Build history of the part. All positions in model axes, mm. A direction names the side the tool comes from. Give positions to 0.01 mm unless a question says otherwise; leave off trailing zeros. Order: outer loops, then holes, each group sorted by start corner. A loop starts at its lowest first (then second) coordinate and runs counter-clockwise, first axis right, second up. Notation, with made-up numbers: (1, 34.5) - (19, 34.5) arc R15 cw to (19, 57.5) - close; hole circle Ø6 at (79, -32). An arc over 180 degrees is marked (long way). Answer in a Markdown table with one row per item.
```python
from build123d import *

# Parameters (mm, degrees)
BOSS_EXTRUDE1_DEPTH = 206
SKETCH2_W           = 10
SKETCH2_H           = 6
BOSS_EXTRUDE2_DEPTH = 10
CUT_EXTRUDE1_REACH  = 202
SKETCH3_R           = 1.5
CUT_EXTRUDE2_REACH  = 33.335
SKETCH4_R           = 2
CUT_EXTRUDE3_REACH  = 33.335
SKETCH5_R           = 1.5
CUT_EXTRUDE4_REACH  = 33.335
SKETCH6_R           = 1.5
CUT_EXTRUDE5_REACH  = 103.569
SKETCH7_R           = 1.5
CUT_EXTRUDE6_REACH  = 103.569
SKETCH8_R           = 1.5


with BuildPart() as part:
    # Sketch1 → Boss-Extrude1 (new body)
    with BuildSketch(Plane(origin=(0, 0, 0), x_dir=(1, 0, 0), z_dir=(0, 1, 0))):
        Polygon((-40, 0), (40, 0), (63.334523779, 23.334523779), (68.991378029, 17.67766953), (43.313708499, -8), (-43.313708499, -8), (-68.991378029, 17.67766953), (-63.334523779, 23.334523779), align=None)
    extrude(amount=BOSS_EXTRUDE1_DEPTH)

    # Sketch2 → Boss-Extrude2 (add)
    with BuildSketch(Plane(origin=(0, 0, 0), x_dir=(-1, 0, 0), z_dir=(0, 0, -1))):
        with Locations((-29, 197)):
            Rectangle(SKETCH2_W, SKETCH2_H)
        with Locations((29, 197)):
            Rectangle(SKETCH2_W, SKETCH2_H)
    extrude(amount=BOSS_EXTRUDE2_DEPTH)

    # Sketch3 → Cut-Extrude1 (cut, up to next)
    with BuildSketch(Plane(origin=(0, 200, 0), x_dir=(1, 0, 0), z_dir=(0, 1, 0)), mode=Mode.PRIVATE) as cut_extrude1_sk1:
        with Locations((-29, 5)):
            Circle(SKETCH3_R)
    cut_extrude1_tool1 = extrude(cut_extrude1_sk1.sketch, amount=-CUT_EXTRUDE1_REACH, mode=Mode.PRIVATE) & part.part
    add(cut_extrude1_tool1.solids().sort_by_distance((-29, 200, -5))[0], mode=Mode.SUBTRACT)
    # Sketch3 → Cut-Extrude1 (cut, up to next)
    with BuildSketch(Plane(origin=(0, 200, 0), x_dir=(1, 0, 0), z_dir=(0, 1, 0)), mode=Mode.PRIVATE) as cut_extrude1_sk2:
        with Locations((29, 5)):
            Circle(SKETCH3_R)
    cut_extrude1_tool2 = extrude(cut_extrude1_sk2.sketch, amount=-CUT_EXTRUDE1_REACH, mode=Mode.PRIVATE) & part.part
    add(cut_extrude1_tool2.solids().sort_by_distance((29, 200, -5))[0], mode=Mode.SUBTRACT)

    # Sketch4 → Cut-Extrude2 (cut, up to next)
    with BuildSketch(Plane.XY.offset(8), mode=Mode.PRIVATE) as cut_extrude2_sk1:
        with Locations((-14.667053615, 27)):
            Circle(SKETCH4_R)
    cut_extrude2_tool1 = extrude(cut_extrude2_sk1.sketch, amount=-CUT_EXTRUDE2_REACH, mode=Mode.PRIVATE) & part.part
    add(cut_extrude2_tool1.solids().sort_by_distance((-14.667054, 27, 8))[0], mode=Mode.SUBTRACT)
    # Sketch4 → Cut-Extrude2 (cut, up to next)
    with BuildSketch(Plane.XY.offset(8), mode=Mode.PRIVATE) as cut_extrude2_sk2:
        with Locations((11.313708499, 12)):
            Circle(SKETCH4_R)
    cut_extrude2_tool2 = extrude(cut_extrude2_sk2.sketch, amount=-CUT_EXTRUDE2_REACH, mode=Mode.PRIVATE) & part.part
    add(cut_extrude2_tool2.solids().sort_by_distance((11.313708, 12, 8))[0], mode=Mode.SUBTRACT)

    # Sketch5 → Cut-Extrude3 (cut, up to next)
    with BuildSketch(Plane.XY.offset(8), mode=Mode.PRIVATE) as cut_extrude3_sk1:
        with Locations((-7, 76.404082058)):
            Circle(SKETCH5_R)
    cut_extrude3_tool1 = extrude(cut_extrude3_sk1.sketch, amount=-CUT_EXTRUDE3_REACH, mode=Mode.PRIVATE) & part.part
    add(cut_extrude3_tool1.solids().sort_by_distance((-7, 76.404082, 8))[0], mode=Mode.SUBTRACT)
    # Sketch5 → Cut-Extrude3 (cut, up to next)
    with BuildSketch(Plane.XY.offset(8), mode=Mode.PRIVATE) as cut_extrude3_sk2:
        with Locations((7, 76.404082058)):
            Circle(SKETCH5_R)
    cut_extrude3_tool2 = extrude(cut_extrude3_sk2.sketch, amount=-CUT_EXTRUDE3_REACH, mode=Mode.PRIVATE) & part.part
    add(cut_extrude3_tool2.solids().sort_by_distance((7, 76.404082, 8))[0], mode=Mode.SUBTRACT)

    # Sketch6 → Cut-Extrude4 (cut, up to next)
    with BuildSketch(Plane.XY.offset(8), mode=Mode.PRIVATE) as cut_extrude4_sk1:
        with Locations((-25.813708499, 171)):
            Circle(SKETCH6_R)
    cut_extrude4_tool1 = extrude(cut_extrude4_sk1.sketch, amount=-CUT_EXTRUDE4_REACH, mode=Mode.PRIVATE) & part.part
    add(cut_extrude4_tool1.solids().sort_by_distance((-25.813708, 171, 8))[0], mode=Mode.SUBTRACT)
    # Sketch6 → Cut-Extrude4 (cut, up to next)
    with BuildSketch(Plane.XY.offset(8), mode=Mode.PRIVATE) as cut_extrude4_sk2:
        with Locations((25.813708499, 171)):
            Circle(SKETCH6_R)
    cut_extrude4_tool2 = extrude(cut_extrude4_sk2.sketch, amount=-CUT_EXTRUDE4_REACH, mode=Mode.PRIVATE) & part.part
    add(cut_extrude4_tool2.solids().sort_by_distance((25.813708, 171, 8))[0], mode=Mode.SUBTRACT)
    # Sketch6 → Cut-Extrude4 (cut, up to next)
    with BuildSketch(Plane.XY.offset(8), mode=Mode.PRIVATE) as cut_extrude4_sk3:
        with Locations((-25.813708499, 106)):
            Circle(SKETCH6_R)
    cut_extrude4_tool3 = extrude(cut_extrude4_sk3.sketch, amount=-CUT_EXTRUDE4_REACH, mode=Mode.PRIVATE) & part.part
    add(cut_extrude4_tool3.solids().sort_by_distance((-25.813708, 106, 8))[0], mode=Mode.SUBTRACT)
    # Sketch6 → Cut-Extrude4 (cut, up to next)
    with BuildSketch(Plane.XY.offset(8), mode=Mode.PRIVATE) as cut_extrude4_sk4:
        with Locations((25.813708499, 89)):
            Circle(SKETCH6_R)
    cut_extrude4_tool4 = extrude(cut_extrude4_sk4.sketch, amount=-CUT_EXTRUDE4_REACH, mode=Mode.PRIVATE) & part.part
    add(cut_extrude4_tool4.solids().sort_by_distance((25.813708, 89, 8))[0], mode=Mode.SUBTRACT)

    # Sketch7 → Cut-Extrude5 (cut, up to next)
    with BuildSketch(Plane(origin=(-25.656854249, 0, 25.656854249), x_dir=(0.707106781, 0, 0.707106781), z_dir=(-0.707106781, 0, 0.707106781)), mode=Mode.PRIVATE) as cut_extrude5_sk1:
        with Locations((-43.414271247, 171)):
            Circle(SKETCH7_R)
    cut_extrude5_tool1 = extrude(cut_extrude5_sk1.sketch, amount=-CUT_EXTRUDE5_REACH, mode=Mode.PRIVATE) & part.part
    add(cut_extrude5_tool1.solids().sort_by_distance((-56.35538, 171, -5.041671))[0], mode=Mode.SUBTRACT)
    # Sketch7 → Cut-Extrude5 (cut, up to next)
    with BuildSketch(Plane(origin=(-25.656854249, 0, 25.656854249), x_dir=(0.707106781, 0, 0.707106781), z_dir=(-0.707106781, 0, 0.707106781)), mode=Mode.PRIVATE) as cut_extrude5_sk2:
        with Locations((-43.414271247, 81)):
            Circle(SKETCH7_R)
    cut_extrude5_tool2 = extrude(cut_extrude5_sk2.sketch, amount=-CUT_EXTRUDE5_REACH, mode=Mode.PRIVATE) & part.part
    add(cut_extrude5_tool2.solids().sort_by_distance((-56.35538, 81, -5.041671))[0], mode=Mode.SUBTRACT)

    # Sketch8 → Cut-Extrude6 (cut, up to next)
    with BuildSketch(Plane(origin=(25.656854249, 0, 25.656854249), x_dir=(0.707106781, 0, -0.707106781), z_dir=(0.707106781, 0, 0.707106781)), mode=Mode.PRIVATE) as cut_extrude6_sk1:
        with Locations((40.384271247, 171)):
            Circle(SKETCH8_R)
    cut_extrude6_tool1 = extrude(cut_extrude6_sk1.sketch, amount=-CUT_EXTRUDE6_REACH, mode=Mode.PRIVATE) & part.part
    add(cut_extrude6_tool1.solids().sort_by_distance((54.212846, 171, -2.899138))[0], mode=Mode.SUBTRACT)
    # Sketch8 → Cut-Extrude6 (cut, up to next)
    with BuildSketch(Plane(origin=(25.656854249, 0, 25.656854249), x_dir=(0.707106781, 0, -0.707106781), z_dir=(0.707106781, 0, 0.707106781)), mode=Mode.PRIVATE) as cut_extrude6_sk2:
        with Locations((40.384271247, 76)):
            Circle(SKETCH8_R)
    cut_extrude6_tool2 = extrude(cut_extrude6_sk2.sketch, amount=-CUT_EXTRUDE6_REACH, mode=Mode.PRIVATE) & part.part
    add(cut_extrude6_tool2.solids().sort_by_distance((54.212846, 76, -2.899138))[0], mode=Mode.SUBTRACT)


solid = part.part
```
1. Cut at D-D on x = -46.5. Write the cut outline in (y, z).
Check result:
| item | result |
|---|---|
| outline | (0, -6.5) - (206, -6.5) - (206, 4.81) - (0, 4.81) - close |
2. Drop flat-ended pins along their axis: P1, Ø4, axis at y = 35, z = 4, coming from the +X side; P2, Ø10, axis at y = 27, z = 2, coming from the +X side; P3, Ø6.5, axis at x = -14.67, y = 27, coming from the -Z side; P4, Ø3.5, axis at x = 25.81, y = 89, coming from the +Z side. Give the stop position or say it passes through.
Check result:
| item | result |
|---|---|
| P1 | stops at x = 49.31 |
| P2 | stops at x = 54.31 |
| P3 | stops at z = 0 |
| P4 | stops at z = 8 |
3. Cut at A-A on y = 27. Write the cut outline in (x, z), and give its area (3 significant figures).
Check result:
| item | result |
|---|---|
| outline | (-68.99, -17.68) - (-63.33, -23.33) - (-40, 0) - (-16.67, 0) - (-16.67, 8) - (-43.31, 8) - close; (-12.67, 0) - (40, 0) - (63.33, -23.33) - (68.99, -17.68) - (43.31, 8) - (-12.67, 8) - close |
| area | 1,190 mm² |
4. Cut at B-B on y = 55. Write the cut outline in (x, z), and give its area (3 significant figures).
Check result:
| item | result |
|---|---|
| outline | (-68.99, -17.68) - (-63.33, -23.33) - (-40, 0) - (40, 0) - (63.33, -23.33) - (68.99, -17.68) - (43.31, 8) - (-43.31, 8) - close |
| area | 1,220 mm² |
5. Two-plate mould, pull along Y, no slides. Class faces 1 (the face through (51.286, 77.487, -5.55)), 2 (the face through (29, 197, -10)), 3 (the face through (30.2, 194, -3.8)): +Y half, -Y half, draft (parallel to the pull), parting line (faces both ways), or undercut.
Check result:
| item | result |
|---|---|
| face 1 | undercut |
| face 2 | draft |
| face 3 | -Y half |
6. Cut at C-C on z = -15. Write the cut outline in (x, y).
Check result:
| item | result |
|---|---|
| outline | (-66.31, 0) - (-55, 0) - (-55, 206) - (-66.31, 206) - close; (55, 0) - (66.31, 0) - (66.31, 206) - (55, 206) - close |
7. Which spindle directions (+Z, -Z, +X, -X, +Y, -Y) get a long thin tool onto all of the face, cutting with end or side? Do faces 4 (the face through (-24, 197, -5)), 5 (the face through (-53.705, 172.487, -7.969)). Say none if no direction does.
Check result:
| item | result |
|---|---|
| face 4 | -Z, +Y, -Y |
| face 5 | none |
8. Probe line 1 (Z direction, x = 29, y = 197.85); line 2 (Z direction, x = 5.5, y = 187.5); line 3 (Y direction, x = -7, z = 5). List the from-to ranges inside material, lowest first.
Check result:
| item | result |
|---|---|
| line 1 | z = -10 to -6.5, -3.5 to 8 |
| line 2 | z = 0 to 8 |
| line 3 | y = 0 to 74.9, 77.9 to 206 |
